Input: part model. Units: mm. Frame: model coordinates. A direction names the side the tool comes from. Round coordinates to 2 decimals unless told otherwise and drop trailing zeros. Write each loop counter-clockwise with the first axis right and the second up, starting at its lowest first coordinate (ties: lowest second). Pieces come first, ordered by that corner, then holes. Notation, with made-up numbers: (-15.5, -30) -> (26.5, -30) arc R23 ccw to (26.5, 9) -> close; hole circle Ø6 at (34.25, -12.5). An arc over 180 degrees is marked (long way). Use CSV: the item, a comma, the result in double quotes.
```python
from build123d import *

# Parameters (mm, degrees)
BOSS_EXTRUDE1_DEPTH      = 44.45
SKETCH2_W                = 88.9
SKETCH2_H                = 31.75
CUT_EXTRUDE1_DEPTH       = 12.7
CUT_EXTRUDE2_DEPTH       = 70.85
F_1_4_1_DIAMETER_HOLE1_D = 25.4


with BuildPart() as part:
    # Sketch1 → Boss-Extrude1 (new body, symmetric)
    with BuildSketch(Plane.XY):
        Polygon((0, 0), (0, 69.85), (63.5, 69.85), (88.9, 57.15), (152.4, 25.4), (152.4, 0), align=None)
    extrude(amount=BOSS_EXTRUDE1_DEPTH, both=True)

    # Sketch2 → Cut-Extrude1 (cut)
    with BuildSketch(Plane(origin=(0, 69.85, 0), x_dir=(1, 0, 0), z_dir=(0, 1, 0))):
        with Locations((44.45, 3.175)):
            Rectangle(SKETCH2_W, SKETCH2_H)
    extrude(amount=-CUT_EXTRUDE1_DEPTH, mode=Mode.SUBTRACT)

    # Sketch3 → Cut-Extrude2 (cut, through all)
    with BuildSketch(Plane(origin=(0, 0, 0), x_dir=(1, 0, 0), z_dir=(0, 1, 0))):
        Polygon((88.9, -44.45), (152.4, 0), (152.4, -44.45), align=None)
    extrude(amount=CUT_EXTRUDE2_DEPTH, mode=Mode.SUBTRACT)

    # 1/4 (1) Diameter Hole1 (through all)
    with Locations(Plane.XY.offset(44.45)):
        with Locations((38.1, 31.75)):
            Hole(F_1_4_1_DIAMETER_HOLE1_D / 2)


solid = part.part
```
Item 1: Section query A-A on y = 65.5. Return the cut outline in (x, z).
Worked answers:
outline,"(0, -44.45) -> (72.2, -44.45) -> (72.2, -19.05) -> (0, -19.05) -> close; (0, 12.7) -> (72.2, 12.7) -> (72.2, 44.45) -> (0, 44.45) -> close"
Item 2: Section query B-B on x = 38.1. Return the cut outline in (y, z), plus the area to 3 significant figures.
Worked answers:
outline,"(0, -44.45) -> (19.05, -44.45) -> (19.05, 44.45) -> (0, 44.45) -> close; (44.45, -44.45) -> (69.85, -44.45) -> (69.85, -19.05) -> (57.15, -19.05) -> (57.15, 12.7) -> (69.85, 12.7) -> (69.85, 44.45) -> (44.45, 44.45) -> close"
area,"3,550 mm²"
Item 3: Pull-direction query (Y, two-part tool) for faces 1 (the face through (44, 57.15, -3)), 2 (the face through (34, 64, -19.05)), 3 (the face through (48.178, 24.022, -0.622)); classes: +Y half, -Y half, draft (parallel to the pull), parting line (faces both ways), or undercut.
Worked answers:
face 1,"+Y half"
face 2,"draft"
face 3,"undercut"
Item 4: Set-up query: faces 4 (the face through (34, 64, 12.7)), 5 (the face through (77, 28, -44.45)). Return all of +Z, -Z, +X, -X, +Y, -Y with unobstructed straight access to the full face (end or side cutting, diameter ignored); none if empty.
Worked answers:
face 4,"+X, -X, +Y"
face 5,"-Z, +X, -X, +Y, -Y"
Item 5: Line query: line 1 (Z direction, x = 23.5, y = 58); line 2 (Y direction, x = 38, z = 3); line 3 (Y direction, x = 38.1, z = 22.5). Output: solid intervals per line, ascending.
Worked answers:
line 1,"z = -44.45 to -19.05, 12.7 to 44.45"
line 2,"y = 0 to 19.05, 44.45 to 57.15"
line 3,"y = 0 to 19.05, 44.45 to 69.85"
Item 6: First-contact query: pin 1 Ø6 at (x, y) = (134.5, 9.5) entering from +Z; pin 2 Ø12 at (y, z) = (32.5, -24.5) entering from +X; pin 3 Ø15 at (x, y) = (38.1, 31.75) entering from +Z. Flat tips, straight axial feed; report the tip coordinate or a pass-through.
Worked answers:
pin 1,"stops at z = 14.63"
pin 2,"stops at x = 150.2"
pin 3,"passes through"
Item 7: Section query D-D on x = 76. Return the cut outline in (y, z), plus the area to 3 significant figures.
Worked answers:
outline,"(0, -44.45) -> (63.6, -44.45) -> (63.6, -19.05) -> (57.15, -19.05) -> (57.15, 12.7) -> (63.6, 12.7) -> (63.6, 44.45) -> (0, 44.45) -> close"
area,"5,450 mm²"
Item 8: Section query C-C on z = 17.5. Return the cut outline in (x, y).
Worked answers:
outline,"(0, 0) -> (127.4, 0) -> (127.4, 37.9) -> (63.5, 69.85) -> (0, 69.85) -> close; hole circle Ø25.4 at (38.1, 31.75)"
